Could you check a few things on this model? Use its own coordinates, in mm. A direction names the side the tool comes from. Round coordinates to 2 decimals unless told otherwise and drop trailing zeros. Loops run counter-clockwise (first coordinate to the right, second up) from the corner with the lowest first, then second, coordinate; pieces in that order, holes last.
from build123d import *

# Parameters (mm, degrees)
SKETCH1_W           = 255
SKETCH1_H           = 260
SKETCH1_R           = 60
BOSS_EXTRUDE1_DEPTH = 8
SKETCH2_W           = 70
SKETCH2_H           = 30
SKETCH2_W_2         = 80
BOSS_EXTRUDE2_DEPTH = 60
BOSS_EXTRUDE3_DEPTH = 60
CUT_EXTRUDE1_DEPTH  = 60
CUT_EXTRUDE2_DEPTH  = 60


with BuildPart() as part:
    # Sketch1 → Boss-Extrude1 (new body)
    with BuildSketch(Plane.XY):
        Rectangle(SKETCH1_W, SKETCH1_H)
        with Locations((0, 20)):
            Circle(SKETCH1_R, mode=Mode.SUBTRACT)
    extrude(amount=BOSS_EXTRUDE1_DEPTH)

    # Sketch2 → Boss-Extrude2 (add)
    with BuildSketch(Plane.XY.offset(8)):
        Polygon((0, -130), (157.5, -130), (157.5, -200), (-157.5, -200), (-157.5, -130), align=None)
        with Locations((0, -165)):
            Rectangle(SKETCH2_W, SKETCH2_H, mode=Mode.SUBTRACT)
        with Locations((90, -165)):
            Rectangle(SKETCH2_W_2, SKETCH2_H, mode=Mode.SUBTRACT)
        with Locations((-90, -165)):
            Rectangle(SKETCH2_W_2, SKETCH2_H, mode=Mode.SUBTRACT)
    extrude(amount=-BOSS_EXTRUDE2_DEPTH)

    # Sketch3 → Boss-Extrude3 (add)
    with BuildSketch(Plane(origin=(0, -130, 0), x_dir=(1, 0, 0), z_dir=(0, 1, 0))):
        Polygon((127.5, -8), (157.5, 42), (153.970588235, 44.117647059), (127.5, 0), align=None)
    boss_extrude3 = extrude(amount=BOSS_EXTRUDE3_DEPTH)

    # Sketch4 → Cut-Extrude1 (cut)
    with BuildSketch(Plane(origin=(97.279411765, 0, 58.367647059), x_dir=(0.5144957554275268, 0, -0.8574929257125441), z_dir=(0.8574929257125441, 0, 0.5144957554275268))):
        Polygon((65.598208817, -70), (117.04778436, -130), (117.04778436, -70), align=None)
    extrude(amount=-CUT_EXTRUDE1_DEPTH, mode=Mode.SUBTRACT)

    # Mirror4: Boss-Extrude3 across plane
    add(boss_extrude3.mirror(Plane(origin=(0, 0, 0), x_dir=(0, 0, 1), z_dir=(1, 0, 0))))

    # Sketch5 → Cut-Extrude2 (cut)
    with BuildSketch(Plane(origin=(-97.279411765, 0, 58.367647059), x_dir=(0.514495755427527, 0, 0.857492925712544), z_dir=(-0.857492925712544, 0, 0.514495755427527))):
        Polygon((-65.598208817, -70), (-117.04778436, -130), (-117.04778436, -70), align=None)
    extrude(amount=-CUT_EXTRUDE2_DEPTH, mode=Mode.SUBTRACT)


solid = part.part
Item 1: If we section it at D-D, the plane x = 0: Please give me the cut outline in (y, z), then the cut area to 3 significant figures.
Results list:
outline: (-200, -52) - (-180, -52) - (-180, 8) - (-200, 8) - close; (-150, -52) - (-130, -52) - (-130, 0) - (-40, 0) - (-40, 8) - (-150, 8) - close; (80, 0) - (130, 0) - (130, 8) - (80, 8) - close
area: 3,520 mm2
Item 2: If we section it at C-C, the plane y = 20: Please give me the cut outline in (x, z).
Results list:
outline: (-127.5, 0) - (-60, 0) - (-60, 8) - (-127.5, 8) - close; (60, 0) - (127.5, 0) - (127.5, 8) - (60, 8) - close
Item 3: For faces 1 (the flat face through (-135.038, -113.753, -12.564)), 2 (the flat face through (146, -130, -11)), 3 (the flat face through (35, -165, -22)), which set-ups out of +Z, -Z, +X, -X, +Y, -Y let a thin tool reach every point of the face, with its end or its side?
Results list:
face 1: -Z, +Y
face 2: +Z, +X, +Y
face 3: +Z, -Z
Item 4: If we section it at A-A, the plane x = -122: Please give me the cut outline in (y, z).
Results list:
outline: (-200, -52) - (-180, -52) - (-180, 8) - (-200, 8) - close; (-150, -52) - (-130, -52) - (-130, 0) - (130, 0) - (130, 8) - (-150, 8) - close
Item 5: If I drill on line 1 along X through (y, z) = (-157.5, -25); line 2 along Y through (x, z) = (0, 2); line 3 along Y through (x, z) = (52.5, -46.5), over which ranges is the centre line in solid material (lowest first)?
Results list:
line 1: x = -157.5 to -130, -50 to -35, 35 to 50, 130 to 157.5
line 2: y = -200 to -180, -150 to -40, 80 to 130
line 3: y = -200 to -180, -150 to -130
Item 6: Will these pins go through, and if not, where does the flat tip stop? pin 1 (2 mm diameter, centred on x = 25, y = -38, fed in from -Z); pin 2 (1.8 mm diameter, centred on x = 130, z = 5, fed in from +Y); pin 3 (4 mm diameter, centred on x = 16, z = -36.5, fed in from +Y).
Results list:
pin 1: stops at z = 0
pin 2: stops at y = -70
pin 3: stops at y = -130
Item 7: We'd pull the mould along Y, two halves only. Please class faces 4 (the flat face through (2, -200, -22)), 5 (the flat face through (-91, -180, -22)), 6 (the flat face through (-149, -130, -6)): released by +Y, released by -Y, zero draft, split by the parting line, or undercut.
Results list:
face 4: released by -Y
face 5: undercut
face 6: released by +Y
Item 8: If we section it at B-B, the plane z = -15.5: Please give me the cut outline in (x, y).
Results list:
outline: (-157.5, -200) - (157.5, -200) - (157.5, -130) - (141.6, -130) - (141.6, -93.96) - (136.8, -91.08) - (136.8, -130) - (-136.8, -130) - (-136.8, -91.08) - (-141.6, -93.96) - (-141.6, -130) - (-157.5, -130) - close; hole (-130, -180) - (-50, -180) - (-50, -150) - (-130, -150) - close; hole (-35, -180) - (35, -180) - (35, -150) - (-35, -150) - close; hole (50, -180) - (130, -180) - (130, -150) - (50, -150) - close
